```python
from build123d import *

# Parameters (mm, degrees)
BOSS_EXTRUDE1_DEPTH = 75
SKETCH3_W           = 100
SKETCH3_H           = 382.75
SKETCH3_H_2         = 200
CUT_EXTRUDE1_DEPTH  = 195
SKETCH5_R           = 40
BOSS_EXTRUDE2_DEPTH = 100
SKETCH4_R           = 100
BOSS_EXTRUDE3_DEPTH = 100


with BuildPart() as part:
    # Sketch2 → Boss-Extrude1 (new, symmetric)
    with BuildSketch(Plane.XY):
        with BuildLine():
            Line((120, 1342.75), (192.75, 192.75))
            ThreePointArc((192.75, 192.75), (0, 0), (-192.75, 192.75))
            Line((-192.75, 192.75), (-120, 1342.75))
            ThreePointArc((-120, 1342.75), (0, 1462.75), (120, 1342.75))
        make_face()
    extrude(amount=BOSS_EXTRUDE1_DEPTH, both=True)

    # Sketch3 → Cut-Extrude1 (cut, symmetric)
    with BuildSketch(Plane(origin=(0, 0, 0), x_dir=(0, 0, -1), z_dir=(1, 0, 0))):
        with Locations((0, 191.375)):
            Rectangle(SKETCH3_W, SKETCH3_H)
        with Locations((0, 1362.75)):
            Rectangle(SKETCH3_W, SKETCH3_H_2)
    extrude(amount=CUT_EXTRUDE1_DEPTH, both=True, mode=Mode.SUBTRACT)

    # Sketch5 → Boss-Extrude2 (add)
    with BuildSketch(Plane(origin=(0, 0, 50), x_dir=(-1, 0, 0), z_dir=(0, 0, -1))):
        with Locations(Location((0, 1342.75, 0), (0, 0, 180))):
            Circle(SKETCH5_R)
    extrude(amount=BOSS_EXTRUDE2_DEPTH)

    # Sketch4 → Boss-Extrude3 (add)
    with BuildSketch(Plane(origin=(0, 0, 50), x_dir=(-1, 0, 0), z_dir=(0, 0, -1))):
        with Locations(Location((0, 192.75, 0), (0, 0, 180))):
            Circle(SKETCH4_R)
    extrude(amount=BOSS_EXTRUDE3_DEPTH)


solid = part.part
```
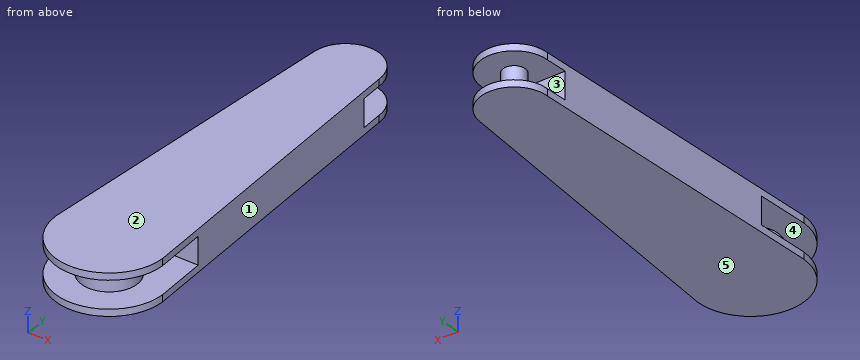
Read the model definition and answer for the solid it produces. Units are mm, in the model's axes. Face numbers are marked on the shaded views. A direction names the side the tool comes from. Coordinates: 2 decimals unless noted, no trailing zeros. Loops run counter-clockwise (first coordinate to the right, second up) from the corner with the lowest first, then second, coordinate; pieces in that order, holes last. Notation, with made-up numbers: (37.5, -19.5) - (48.5, -19.5) arc R23 ccw to (48.5, -11.5) - close; hole circle Ø5 at (-10, 27). An arc over 180 degrees is marked (long way). Answer in a Markdown table with one row per item.
1. Determine the mould class of the marked faces 1, 2 and 3 for opening direction Y: +Y half, -Y half, draft (parallel to the pull), parting line (faces both ways), or undercut.
Conclusion:
| item | result |
|---|---|
| face 1 | +Y half |
| face 2 | draft |
| face 3 | undercut |
2. Given pin 1 (10 mm diameter, centred on y = 369.5, z = -42.5, fed in from -X); pin 2 (5 mm diameter, centred on y = 603, z = -43.5, fed in from +X); pin 3 (3 mm diameter, centred on x = -81, z = 7, fed in from -Y); pin 4 (4 mm diameter, centred on y = 543, z = 55.5, fed in from -X), each flat-ended and moving along its own axis, determine where each tip first touches the part or whether it passes through.
Conclusion:
| item | result |
|---|---|
| pin 1 | passes through |
| pin 2 | stops at x = 166.96 |
| pin 3 | stops at y = 132.09 |
| pin 4 | stops at x = -170.72 |
3. Find section B-B, the plane z = -4. Write down the section's boundary in (x, y).
Conclusion:
| item | result |
|---|---|
| outline | (-180.73, 382.75) - (180.73, 382.75) - (125.06, 1262.75) - (-125.06, 1262.75) - close; circle Ø200 at (0, 192.75); circle Ø80 at (0, 1342.75) |
4. Which of the six approach directions +Z, -Z, +X, -X, +Y, -Y give full straight-line access (tool end or side, diameter ignored) to the marked faces 4 and 5?
Conclusion:
| item | result |
|---|---|
| face 4 | none |
| face 5 | -Z, +X, -X, +Y, -Y |
5. Find section C-C, the plane x = -62. Write down the section's boundary in (y, z), then the cut area to 3 significant figures.
Conclusion:
| item | result |
|---|---|
| outline | (10.24, -75) - (1445.49, -75) - (1445.49, -50) - (1262.75, -50) - (1262.75, 50) - (1445.49, 50) - (1445.49, 75) - (10.24, 75) - (10.24, 50) - (114.29, 50) - (114.29, -50) - (10.24, -50) - close; hole (271.21, -50) - (382.75, -50) - (382.75, 50) - (271.21, 50) - close |
| area | 175,000 mm² |
6. Straight lines are drawn through the part: line 1 (Z direction, x = 142, y = 179.5); line 2 (Y direction, x = -71, z = -23); line 3 (Y direction, x = -8.5, z = -6). For each, find the intervals that lie inside material, in ascending order.
Conclusion:
| item | result |
|---|---|
| line 1 | z = -75 to -50, 50 to 75 |
| line 2 | y = 122.33 to 263.17, 382.75 to 1262.75 |
| line 3 | y = 93.11 to 292.39, 382.75 to 1262.75, 1303.66 to 1381.84 |
7. Find section A-A, the plane x = 0. Write down the section's boundary in (y, z).
Conclusion:
| item | result |
|---|---|
| outline | (0, -75) - (1462.75, -75) - (1462.75, -50) - (1382.75, -50) - (1382.75, 50) - (1462.75, 50) - (1462.75, 75) - (0, 75) - (0, 50) - (92.75, 50) - (92.75, -50) - (0, -50) - close; hole (292.75, -50) - (382.75, -50) - (382.75, 50) - (292.75, 50) - close; hole (1262.75, -50) - (1302.75, -50) - (1302.75, 50) - (1262.75, 50) - close |
8. Find section D-D, the plane y = 153. Write down the section's boundary in (x, z).
Conclusion:
| item | result |
|---|---|
| outline | (-188.61, -75) - (188.61, -75) - (188.61, -50) - (91.76, -50) - (91.76, 50) - (188.61, 50) - (188.61, 75) - (-188.61, 75) - (-188.61, 50) - (-91.76, 50) - (-91.76, -50) - (-188.61, -50) - close |
